Build history of the part. All positions in model axes, mm. A direction names the side the tool comes from. Round coordinates to 2 decimals unless told otherwise and drop trailing zeros. Write each loop counter-clockwise with the first axis right and the second up, starting at its lowest first coordinate (ties: lowest second). Pieces come first, ordered by that corner, then holes.
1) Pull direction Z, two halves, no side cores. Call faces 1 (the flat face through (-51, 18, 61)), 2 (the flat face through (-67.716, 15.465, 67.558)), 3 (the flat face through (50.437, 10.112, -59.064)), 4 (the flat face through (50.437, 10.112, 59.064)): +Z half, -Z half, draft (parallel to the pull), parting line (faces both ways), or undercut.
2) Saw through at B-B (z = -0.5). Write the cut outline in (x, y), plus the area to 3 significant figures.
3) Flat gauge pins, fed straight in: pin 1 (1 mm diameter, centred on y = 2, z = -19, fed in from -X); pin 2 (5 mm diameter, centred on x = -16.5, y = 2.5, fed in from -Z); pin 3 (2 mm diameter, centred on y = 11.5, z = -42, fed in from +X). Where does each tip first touch, or does it go through?
4) Saw through at A-A (y = 7.5). State how many separate pieces and enclosed holes the cut face has, plus the area to 3 significant figures.
5) Wall check: probe 1 along X at (y, z) = (11, 61.5); probe 2 along Z at (x, y) = (-59, 10); probe 3 along X at (y, z) = (5, -44). Give the ranges that are in metal, low to high.
6) Which spindle directions (+Z, -Z, +X, -X, +Y, -Y) get a long thin tool onto all of the face, cutting with end or side? Do faces 5 (the flat face through (63.56, 1.01, -63.51)), 6 (the flat face through (-56, 2, -56)), 7 (the flat face through (49.779, 8.874, -61.092)), 8 (the flat face through (49.779, 8.874, 61.092)). Say none if no direction does.
7) Saw through at C-C (x = -24). Write the cut outline in (y, z).
from build123d import *

# Parameters (mm, degrees)
SKETCH1_W            = 120
SKETCH1_H            = 120
BOSS_EXTRUDE1_DEPTH  = 2
BOSS_EXTRUDE2_DEPTH  = 13
MIRROR2_COPY_1_DEPTH = 13
CUT_EXTRUDE1_DEPTH   = 16.5
MIRROR4_COPY_1_DEPTH = 16.5
BOSS_EXTRUDE3_DEPTH  = 5
CUT_EXTRUDE2_DEPTH   = 6
MIRROR6_COPY_1_DEPTH = 5
MIRROR6_COPY_2_DEPTH = 6
FILLET1_R            = 2
FILLET2_R            = 2
FILLET3_R            = 2
FILLET4_R            = 2


with BuildPart() as part:
    # Sketch1 → Boss-Extrude1 (new body)
    with BuildSketch(Plane(origin=(0, 0, 0), x_dir=(1, 0, 0), z_dir=(0, 1, 0))):
        Polygon((-59.292893219, -70.606601718), (-48.686291501, -60), (-60, -60), (-60, -48.686291501), (-70.606601718, -59.292893219), align=None)
        Polygon((-70.606601718, 59.292893219), (-60, 48.686291501), (-60, 60), (-48.686291501, 60), (-59.292893219, 70.606601718), align=None)
        Rectangle(SKETCH1_W, SKETCH1_H)
        Polygon((60, 60), (60, 48.686291501), (70.606601718, 59.292893219), (59.292893219, 70.606601718), (48.686291501, 60), align=None)
        Polygon((60, -48.686291501), (60, -60), (48.686291501, -60), (59.292893219, -70.606601718), (70.606601718, -59.292893219), align=None)
    extrude(amount=BOSS_EXTRUDE1_DEPTH)

    # Sketch2 → Boss-Extrude2 (add)
    with BuildSketch(Plane(origin=(0, 0, 0), x_dir=(1, 0, 0), z_dir=(0, 1, 0))):
        Polygon((59.292893219, -70.606601718), (70.606601718, -59.292893219), (69.192388155, -57.878679656), (52.787510832, -41.473802333), (48.544870145, -37.231161646), (37.231161646, -48.544870145), (41.473802333, -52.787510832), (57.878679656, -69.192388155), align=None)
        Polygon((59.222182541, -67.848885271), (67.848885271, -59.222182541), (51.444007948, -42.817305217), (42.817305217, -51.444007948), align=None, mode=Mode.SUBTRACT)
    boss_extrude2 = extrude(amount=BOSS_EXTRUDE2_DEPTH)

    # Mirror1: Boss-Extrude2 across plane
    add(boss_extrude2.mirror(Plane(origin=(0, 0, 0), x_dir=(0, 0, 1), z_dir=(1, 0, 0))))

    # Mirror2: Boss-Extrude2 across plane
    add(boss_extrude2.mirror(Plane.XY))

    # Mirror2 copy 1 sketch → Mirror2 copy 1 (add)
    with BuildSketch(Plane(origin=(0, 0, 0), x_dir=(-1, 0, 0), z_dir=(0, 1, 0))):
        Polygon((59.292893219, -70.606601718), (70.606601718, -59.292893219), (69.192388155, -57.878679656), (52.787510832, -41.473802333), (48.544870145, -37.231161646), (37.231161646, -48.544870145), (41.473802333, -52.787510832), (57.878679656, -69.192388155), align=None)
        Polygon((59.222182541, -67.848885271), (67.848885271, -59.222182541), (51.444007948, -42.817305217), (42.817305217, -51.444007948), align=None, mode=Mode.SUBTRACT)
    extrude(amount=MIRROR2_COPY_1_DEPTH)

    # Sketch3 → Cut-Extrude1 (cut)
    with BuildSketch(Plane(origin=(0, 13, 0), x_dir=(1, 0, 0), z_dir=(0, 1, 0))):
        Polygon((61.944543648, -65.126524164), (63.358757211, -66.540737726), (66.540737726, -63.358757211), (65.126524164, -61.944543648), align=None)
    cut_extrude1 = extrude(amount=-CUT_EXTRUDE1_DEPTH, mode=Mode.SUBTRACT)

    # Mirror3: Cut-Extrude1 across plane
    add(cut_extrude1.mirror(Plane(origin=(0, 0, 0), x_dir=(0, 0, 1), z_dir=(1, 0, 0))), mode=Mode.SUBTRACT)

    # Mirror4: Cut-Extrude1 across plane
    add(cut_extrude1.mirror(Plane.XY), mode=Mode.SUBTRACT)

    # Mirror4 copy 1 sketch → Mirror4 copy 1 (cut)
    with BuildSketch(Plane(origin=(0, 13, 0), x_dir=(-1, 0, 0), z_dir=(0, 1, 0))):
        Polygon((61.944543648, -65.126524164), (63.358757211, -66.540737726), (66.540737726, -63.358757211), (65.126524164, -61.944543648), align=None)
    extrude(amount=-MIRROR4_COPY_1_DEPTH, mode=Mode.SUBTRACT)

    # Sketch4 → Boss-Extrude3 (add)
    with BuildSketch(Plane(origin=(0, 13, 0), x_dir=(1, 0, 0), z_dir=(0, 1, 0))):
        Polygon((37.231161646, 48.544870145), (48.544870145, 37.231161646), (73.293607486, 61.979898987), (61.979898987, 73.293607486), align=None)
    boss_extrude3 = extrude(amount=BOSS_EXTRUDE3_DEPTH)

    # Sketch7 → Cut-Extrude2 (cut)
    with BuildSketch(Plane(origin=(0, 18, 0), x_dir=(1, 0, 0), z_dir=(0, 1, 0))):
        Polygon((42.817305217, 51.444007948), (51.444007948, 42.817305217), (67.848885271, 59.222182541), (59.222182541, 67.848885271), align=None)
    cut_extrude2 = extrude(amount=-CUT_EXTRUDE2_DEPTH, mode=Mode.SUBTRACT)

    # Mirror5: Boss-Extrude3, Cut-Extrude2 across plane
    add(boss_extrude3.mirror(Plane.XY))
    add(cut_extrude2.mirror(Plane.XY), mode=Mode.SUBTRACT)

    # Mirror6: Boss-Extrude3, Cut-Extrude2 across plane
    add(boss_extrude3.mirror(Plane(origin=(0, 0, 0), x_dir=(0, 0, 1), z_dir=(1, 0, 0))))
    add(cut_extrude2.mirror(Plane(origin=(0, 0, 0), x_dir=(0, 0, 1), z_dir=(1, 0, 0))), mode=Mode.SUBTRACT)

    # Mirror6 copy 1 sketch → Mirror6 copy 1 (add)
    with BuildSketch(Plane(origin=(0, 13, 0), x_dir=(-1, 0, 0), z_dir=(0, 1, 0))):
        Polygon((37.231161646, 48.544870145), (48.544870145, 37.231161646), (73.293607486, 61.979898987), (61.979898987, 73.293607486), align=None)
    extrude(amount=MIRROR6_COPY_1_DEPTH)

    # Mirror6 copy 2 sketch → Mirror6 copy 2 (cut)
    with BuildSketch(Plane(origin=(0, 18, 0), x_dir=(-1, 0, 0), z_dir=(0, 1, 0))):
        Polygon((42.817305217, 51.444007948), (51.444007948, 42.817305217), (67.848885271, 59.222182541), (59.222182541, 67.848885271), align=None)
    extrude(amount=-MIRROR6_COPY_2_DEPTH, mode=Mode.SUBTRACT)

    # Fillet1
    fillet1_edges = [part.edges().sort_by_distance(p)[0] for p in [
        (-47.130656582, 18, -47.130656582),
    ]]
    fillet(fillet1_edges, radius=FILLET1_R)

    # Fillet2
    fillet2_edges = [part.edges().sort_by_distance(p)[0] for p in [
        (-47.130656582, 18, 47.130656582),
    ]]
    fillet(fillet2_edges, radius=FILLET2_R)

    # Fillet3
    fillet3_edges = [part.edges().sort_by_distance(p)[0] for p in [
        (47.130656582, 18, -47.130656582),
    ]]
    fillet(fillet3_edges, radius=FILLET3_R)

    # Fillet4
    fillet4_edges = [part.edges().sort_by_distance(p)[0] for p in [
        (47.130656582, 18, 47.130656582),
    ]]
    fillet(fillet4_edges, radius=FILLET4_R)


solid = part.part
Evaluation:
1. face 1: draft
1. face 2: +Z half
1. face 3: undercut
1. face 4: undercut
2. outline: (-60, 0) - (60, 0) - (60, 2) - (-60, 2) - close
2. area: 240 mm2
3. pin 1: stops at x = -60
3. pin 2: stops at z = -60
3. pin 3: stops at x = 54.31
4. separate pieces: 4
4. enclosed holes: 0
4. area: 829 mm2
5. probe 1: x = -68.4 to -65.57, -52.87 to -50.19, 50.19 to 52.87, 65.57 to 68.4
5. probe 2: z = -70.31 to -67.63, -50.37 to -47.69, 47.69 to 50.37, 67.63 to 70.31
5. probe 3: x = -55.31 to -52.63, -50.26 to -41.78, 41.78 to 50.26, 52.63 to 55.31
6. face 5: -Y
6. face 6: +Y
6. face 7: -Z, +Y
6. face 8: +Z, +Y
7. outline: (0, -60) - (2, -60) - (2, 60) - (0, 60) - close
